The model under review builds one solid part; all positions refer to its coordinate system, in mm. Face numbers are marked on the shaded views. A direction names the side the tool comes from. Coordinates: 2 decimals unless noted, no trailing zeros. Loops run counter-clockwise (first coordinate to the right, second up) from the corner with the lowest first, then second, coordinate; pieces in that order, holes last. Notation, with made-up numbers: M 55,88 L 104,88 A32 cw 104,122 Z; hole C -29.5,25.25 d2. An arc over 180 degrees is marked long. Return JSON: item names as keys, results as strings.
```python
from build123d import *

# Parameters (mm, degrees)
F0_W     = 12.9794
F0_H     = 25.908
F1_DEPTH = 25.4
F2_W     = 42.2184414506
F2_H     = 12.9794
F3_DEPTH = 12.7
F4_W     = 50.8
F4_H     = 10.4306445336
F5_DEPTH = 50.8
F6_R     = 12.7
F7_DEPTH = 10.4316445336
F8_R     = 25.4
F9_R     = 25.39999


# Not quite as in the source:
# - a fillet or chamfer is up to 0.001 mm smaller than in the source, because OpenCascade refuses the exact size


with BuildPart() as f1:
    # F0 (on Right) → F1 (new body, symmetric)
    with BuildSketch(Plane.YZ):
        with Locations((35.6550812721, 2.5243262509)):
            Rectangle(F0_W, F0_H)
    extrude(amount=F1_DEPTH, both=True)

    # F2 (on face) → F3 (join)
    with BuildSketch(Plane.XY.offset(15.4783262509)):
        with Locations((4.2907792747, 35.6550812721)):
            Rectangle(F2_W, F2_H)
    extrude(amount=F3_DEPTH)

    # F4 (on face) → F5 (join)
    with BuildSketch(Plane.XZ.offset(-29.1653812721)):
        with Locations((0, -5.2143514823)):
            Rectangle(F4_W, F4_H)
    extrude(amount=F5_DEPTH)

    # F6 (on face) → F7 (cut, through all)
    with BuildSketch(Plane.XY.offset(0.0009707845)):
        with Locations((0, 3.7653812721)):
            Circle(F6_R)
    extrude(amount=-F7_DEPTH, mode=Mode.SUBTRACT)

    # F8
    f8_edges = [f1.edges().sort_by_distance(p)[0] for p in [
        (-25.4, -21.634619, -5.214351),
    ]]
    fillet(f8_edges, radius=F8_R)

    # F9 (radius 25.4 in the source; OpenCascade refuses exactly that, so slightly less here)
    f9_edges = [f1.edges().sort_by_distance(p)[0] for p in [
        (25.4, -21.634619, -5.214351),
    ]]
    fillet(f9_edges, radius=F9_R)


solid = f1.part
```
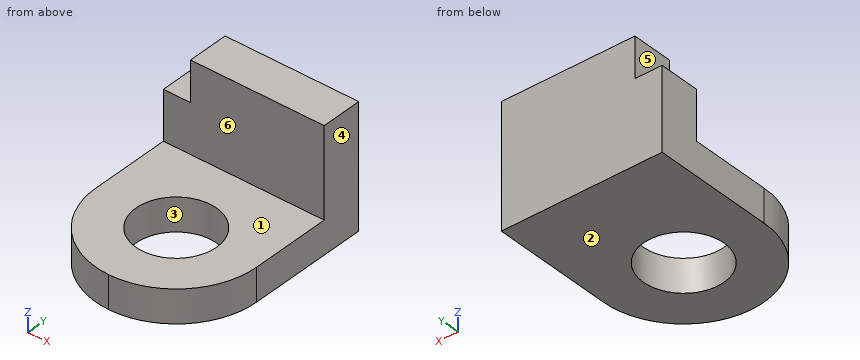
1. Add section A-A on x = -8. Give the boundary of the cut face in (y, z), plus the area to 3 significant figures.
Check values:
{"outline": "M -20.34,-10.43 L -6.1,-10.43 L -6.1,0 L -20.34,0 Z; M 13.63,-10.43 L 42.14,-10.43 L 42.14,28.18 L 29.17,28.18 L 29.17,0 L 13.63,0 Z", "area": "812 mm²"}
2. To check wall thickness, follow line 1 (Y direction, x = 0, z = -7.75); line 2 (Y direction, x = 14, z = 18.5); line 3 (Z direction, x = -22, y = 4.5). State the ranges of each line that lie inside material, in increasing order.
Check values:
{"line 1": "-21.63 to -8.93, 16.47 to 42.14", "line 2": "29.17 to 42.14", "line 3": "-10.43 to 0"}
3. Machinability: for the marked faces 4, 5 and 6, which of the approach directions +Z, -Z, +X, -X, +Y, -Y give a long, thin tool a straight path to every point of the face, cutting with its end or side? Answer none if there is none.
Check values:
{"face 4": "+Z, -Z, +X, +Y, -Y", "face 5": "+Z, -X, +Y, -Y", "face 6": "+Z, +X, -X, -Y"}
4. The part is to be moulded in two halves that separate along Z. For the marked faces 1, 2 and 3, say which applies: released by +Z, released by -Z, zero draft, split by the parting line, or undercut.
Check values:
{"face 1": "released by +Z", "face 2": "released by -Z", "face 3": "zero draft"}
5. Add section B-B on y = -2. Give the boundary of the cut face in (x, z).
Check values:
{"outline": "M -24.74,-10.43 L -11.32,-10.43 L -11.32,0 L -24.74,0 Z; M 11.32,-10.43 L 24.74,-10.43 L 24.74,0 L 11.32,0 Z"}
6. Add section D-D on y = 36.5. Give the boundary of the cut face in (x, z), plus the area to 3 significant figures.
Check values:
{"outline": "M -25.4,-10.43 L 25.4,-10.43 L 25.4,28.18 L -16.82,28.18 L -16.82,15.48 L -25.4,15.48 Z", "area": "1,850 mm²"}
7. Insertion check: pin 1 Ø22.5 at (x, z) = (-10.5, 19) entering from -Y; pin 2 Ø10 at (x, y) = (6.5, -6.5) entering from -Z; pin 3 Ø12 at (y, z) = (-4.5, -5.5) entering from +X; pin 4 Ø1 at (x, y) = (-7, -5.5) entering from +Z. Each pin has a flat end and moves straight along its axis. Give the tip position at first contact, or say it passes through.
Check values:
{"pin 1": "y = 29.17", "pin 2": "z = -10.43", "pin 3": "x = 25.3", "pin 4": "through"}
